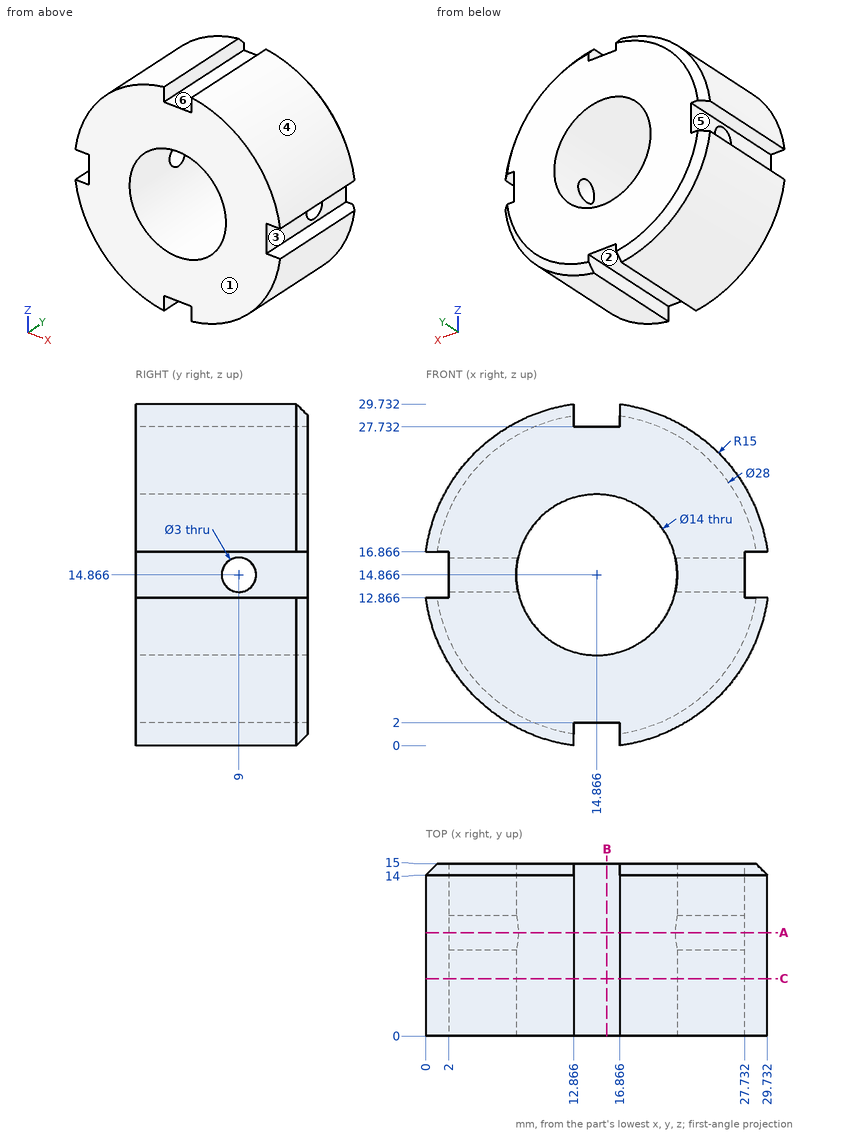
Study the drawing (mm; zero at the part's minimum x, y, z) and answer. A direction names the side the tool comes from. Coordinates: 2 decimals unless noted, no trailing zeros. Loops run counter-clockwise (first coordinate to the right, second up) from the corner with the lowest first, then second, coordinate; pieces in that order, holes last. Notation, with made-up numbers: M 47.25,4.5 L 100.25,4.5 A28 cw 100.25,38.5 Z; hole C 54.5,82 d11. An arc over 180 degrees is marked long. Answer in a Markdown table with one row per item.
1) Find section A-A (y = 9). Determine the outline of the cut face in (x, z), then the cut area to 3 significant figures.
Answers below:
| item | result |
|---|---|
| outline | M 0,12.87 A15 ccw 12.87,0 L 12.87,2 L 16.87,2 L 16.87,0 A15 ccw 29.73,12.87 L 27.73,12.87 L 27.73,13.37 L 21.7,13.37 A7 cw 8.03,13.37 L 2,13.37 L 2,12.87 Z; M 0,16.87 L 2,16.87 L 2,16.37 L 8.03,16.37 A7 cw 21.7,16.37 L 27.73,16.37 L 27.73,16.87 L 29.73,16.87 A15 ccw 16.87,29.73 L 16.87,27.73 L 12.87,27.73 L 12.87,29.73 A15 ccw Z |
| area | 484 mm^2 |
2) Find section B-B (x = 15.75). Determine the outline of the cut face in (y, z).
Answers below:
| item | result |
|---|---|
| outline | M 0,2 L 15,2 L 15,7.92 L 0,7.92 Z; M 0,21.81 L 15,21.81 L 15,27.73 L 0,27.73 Z |
3) Determine the mould class of the marked faces 4, 5 and 6 for opening direction X: released by +X, released by -X, zero draft, split by the parting line, or undercut.
Answers below:
| item | result |
|---|---|
| face 4 | released by +X |
| face 5 | released by -X |
| face 6 | undercut |
4) Which of the six approach directions +Z, -Z, +X, -X, +Y, -Y give full straight-line access (tool end or side, diameter ignored) to the marked faces 1, 2 and 3?
Answers below:
| item | result |
|---|---|
| face 1 | +Z, -Z, +X, -X, -Y |
| face 2 | -Z, +Y, -Y |
| face 3 | +X, +Y, -Y |
5) Find the intervals of material crossed by probe 1 along Z at (x, y) = (15, 14) (1 decimal); probe 2 along Z at (x, y) = (10.75, 1); probe 3 along X at (y, z) = (5.25, 17.5), in increasing order.
Answers below:
| item | result |
|---|---|
| probe 1 | 2 to 7.9, 21.9 to 27.7 |
| probe 2 | 0.44 to 9.2, 20.53 to 29.29 |
| probe 3 | 0.1 to 8.38, 21.35 to 29.63 |
6) Find section C-C (y = 5). Determine the outline of the cut face in (x, z).
Answers below:
| item | result |
|---|---|
| outline | M 0,12.87 A15 ccw 12.87,0 L 12.87,2 L 16.87,2 L 16.87,0 A15 ccw 29.73,12.87 L 27.73,12.87 L 27.73,16.87 L 29.73,16.87 A15 ccw 16.87,29.73 L 16.87,27.73 L 12.87,27.73 L 12.87,29.73 A15 ccw 0,16.87 L 2,16.87 L 2,12.87 Z; hole C 14.87,14.87 d14 |
7) Given pin 1 (1.2 mm diameter, centred on x = 14.5, y = 7, fed in from -Z); pin 2 (3 mm diameter, centred on y = 12, z = 8.5, fed in from -X); pin 3 (0.6 mm diameter, centred on y = 4, z = 29, fed in from +X) (1 decimal), each flat-ended and moving along its own axis, determine where each tip first touches the part or whether it passes through.
Answers below:
| item | result |
|---|---|
| pin 1 | z = 2 |
| pin 2 | x = 0.68 |
| pin 3 | x = 20.7 |
